Here's how the part is built. I have some questions about the finished solid (model axes, mm). A direction names the side the tool comes from. Coordinates: 2 decimals unless noted, no trailing zeros. Order: outer loops, then holes, each group sorted by start corner. A loop starts at its lowest first (then second) coordinate and runs counter-clockwise, first axis right, second up. Notation, with made-up numbers: (-17.5, 24) - (5.5, 24) arc R31 cw to (5.5, 61) - close; hole circle Ø6 at (22.5, 28). An arc over 180 degrees is marked (long way). Answer in a Markdown table with one row per item. Add a question column.
Item 1: If I drill on line 1 along X through (y, z) = (-4.2, 0); line 2 along Y through (x, z) = (-1.25, 0); line 3 along Y through (x, z) = (-3, 2), over which ranges is the centre line in solid material (lowest first)? Write a range as from..to.
Item 2: Will these pins go through, and if not, where does the flat tip stop? pin 1 Ø1.5 at (x, y) = (-3, -1.5) entering from +Z; pin 2 Ø2.5 at (x, z) = (1.5, -0.5) entering from +Y; pin 3 Ø0.6 at (x, z) = (3, -1.5) entering from -Y; pin 4 Ø2 at (x, z) = (2.5, 2.5) entering from -Y.
Item 3: On a 3-axis mill with a long thin cutter (end or side, diameter ignored), from which of +Z, -Z, +X, -X, +Y, -Y can I reach the whole of each face in a straight line? I mean faces 1 (the cylindrical face through (-0.45, 6.75, -1.43)), 2 (the flat face through (3.6, 0, -2.1)), 3 (the flat face through (0, 0, 4.2)), 4 (the cylindrical face through (0.9, -4.22, -2.86)). Say none if no direction works.
Item 4: I want a section at A-A (y = -3.25). Please give me the cut outline in (x, z), plus the area to 3 significant figures.
Item 5: Thinking about a two-plate mould opening in Y: for faces 5 (the flat face through (-2.028, 1.232, 3.448)), 6 (the flat face through (-2, -7, 0)), 7 (the cylindrical face through (-0.976, 6.246, 0.217)), which applies, +Y half, -Y half, draft (parallel to the pull), parting line (faces both ways), or undercut?
```python
from build123d import *

# Parameters (mm, degrees)
BOSS_EXTRUDE5_DEPTH  = 2.5
SKETCH6_R            = 4
BOSS_EXTRUDE6_DEPTH  = 2
SKETCH7_R            = 3
BOSS_EXTRUDE7_DEPTH  = 5
SKETCH8_R            = 1.5
CUT_EXTRUDE1_DEPTH   = 4
SKETCH9_R            = 1.5
BOSS_EXTRUDE8_DEPTH  = 3.5
SKETCH10_R           = 3.5
BOSS_EXTRUDE9_DEPTH  = 0.5
SKETCH11_R           = 3.5
BOSS_EXTRUDE10_DEPTH = 1
BOSS_EXTRUDE10_TAPER = 45
BOSS_EXTRUDE11_START = -4
SKETCH12_R           = 1.5
BOSS_EXTRUDE11_DEPTH = 11.5
CUT_EXTRUDE2_START   = -13
SKETCH13_R           = 1.5
SKETCH13_R_2         = 1
CUT_EXTRUDE2_DEPTH   = 0.5
CUT_EXTRUDE3_START   = -0.5
SKETCH14_R           = 1.5
SKETCH14_R_2         = 1
CUT_EXTRUDE3_DEPTH   = 0.5
CHAMFER1_SIZE        = 0.288675135
CHAMFER1_SIZE2       = 0.5
CHAMFER2_SIZE        = 0.5


with BuildPart() as part:
    # Sketch5 → Boss-Extrude5 (new body)
    with BuildSketch(Plane(origin=(0, 0, 0), x_dir=(1, 0, 0), z_dir=(0, 1, 0))):
        Polygon((-4, 2.309401077), (-4, -2.309401077), (0, -4.618802154), (4, -2.309401077), (4, 2.309401077), (0, 4.618802154), align=None)
    extrude(amount=BOSS_EXTRUDE5_DEPTH)

    # Sketch6 → Boss-Extrude6 (add)
    with BuildSketch(Plane.XZ):
        with Locations(Location((0, 0, 0), (0, 0, 60))):
            Circle(SKETCH6_R)
    extrude(amount=BOSS_EXTRUDE6_DEPTH)

    # Sketch7 → Boss-Extrude7 (add)
    with BuildSketch(Plane.XZ.offset(2)):
        with Locations(Location((0, 0, 0), (0, 0, 270))):
            Circle(SKETCH7_R)
    extrude(amount=BOSS_EXTRUDE7_DEPTH)

    # Sketch8 → Cut-Extrude1 (cut)
    with BuildSketch(Plane.XZ.offset(7)):
        with Locations(Location((0, 0, 0), (0, 0, 270))):
            Circle(SKETCH8_R)
    extrude(amount=-CUT_EXTRUDE1_DEPTH, mode=Mode.SUBTRACT)

    # Sketch9 → Boss-Extrude8 (add)
    with BuildSketch(Plane(origin=(0, 2.5, 0), x_dir=(1, 0, 0), z_dir=(0, 1, 0))):
        with Locations(Location((0, 0, 0), (0, 0, 90))):
            Circle(SKETCH9_R)
    extrude(amount=BOSS_EXTRUDE8_DEPTH)

    # Sketch10 → Boss-Extrude9 (add)
    with BuildSketch(Plane(origin=(0, 2.5, 0), x_dir=(1, 0, 0), z_dir=(0, 1, 0))):
        with Locations(Location((0, 0, 0), (0, 0, 270))):
            Circle(SKETCH10_R)
    extrude(amount=BOSS_EXTRUDE9_DEPTH)

    # Sketch11 → Boss-Extrude10 (add)
    with BuildSketch(Plane(origin=(0, 3, 0), x_dir=(1, 0, 0), z_dir=(0, 1, 0))):
        with Locations(Location((0, 0, 0), (0, 0, 270))):
            Circle(SKETCH11_R)
    extrude(amount=BOSS_EXTRUDE10_DEPTH, taper=BOSS_EXTRUDE10_TAPER)

    # Sketch12 → Boss-Extrude11 (add)
    with BuildSketch(Plane.XZ.offset(7).offset(BOSS_EXTRUDE11_START)):
        with Locations(Location((0, 0, 0), (0, 0, 270))):
            Circle(SKETCH12_R)
    extrude(amount=-BOSS_EXTRUDE11_DEPTH)

    # Sketch13 → Cut-Extrude2 (cut)
    with BuildSketch(Plane.XZ.offset(7).offset(CUT_EXTRUDE2_START)):
        with Locations(Location((0, 0, 0), (0, 0, 270))):
            Circle(SKETCH13_R)
        with Locations(Location((0, 0, 0), (0, 0, 270))):
            Circle(SKETCH13_R_2, mode=Mode.SUBTRACT)
    extrude(amount=-CUT_EXTRUDE2_DEPTH, mode=Mode.SUBTRACT)

    # Sketch14 → Cut-Extrude3 (cut)
    with BuildSketch(Plane.XZ.offset(-6.5).offset(CUT_EXTRUDE3_START)):
        with Locations(Location((0, 0, 0), (0, 0, 270))):
            Circle(SKETCH14_R)
        with Locations(Location((0, 0, 0), (0, 0, 270))):
            Circle(SKETCH14_R_2, mode=Mode.SUBTRACT)
    extrude(amount=-CUT_EXTRUDE3_DEPTH, mode=Mode.SUBTRACT)

    # Chamfer1
    chamfer1_edges = [part.edges().sort_by_distance(p)[0] for p in [
        (0, 8.5, 1.5),
    ]]
    chamfer1_side = [part.faces().sort_by_distance(p)[0] for p in [
        (0, 8, 1.5),
    ]]
    chamfer(chamfer1_edges, length=CHAMFER1_SIZE, length2=CHAMFER1_SIZE2, reference=chamfer1_side[0])

    # Chamfer2
    chamfer2_edges = [part.edges().sort_by_distance(p)[0] for p in [
        (0, -7, 3),
    ]]
    chamfer(chamfer2_edges, length=CHAMFER2_SIZE)


solid = part.part
```
Values follow:
| question | item | result |
|---|---|---|
| 1 | line 1 | x = -3..-1.5, 1.5..3 |
| 1 | line 2 | y = -3..6, 6.5..7, 7.5..8.36 |
| 1 | line 3 | y = -2..2.5 |
| 2 | pin 1 | stops at z = 3.31 |
| 2 | pin 2 | stops at y = 8.5 |
| 2 | pin 3 | stops at y = -2 |
| 2 | pin 4 | stops at y = -6.96 |
| 3 | face 1 | +Y |
| 3 | face 2 | -Z, +X, -Y |
| 3 | face 3 | +Z, -Y |
| 3 | face 4 | -Y |
| 4 | outline | circle Ø6 at (0, 0); hole circle Ø3 at (0, 0) |
| 4 | area | 21.2 mm^2 |
| 5 | face 5 | draft |
| 5 | face 6 | -Y half |
| 5 | face 7 | undercut |
